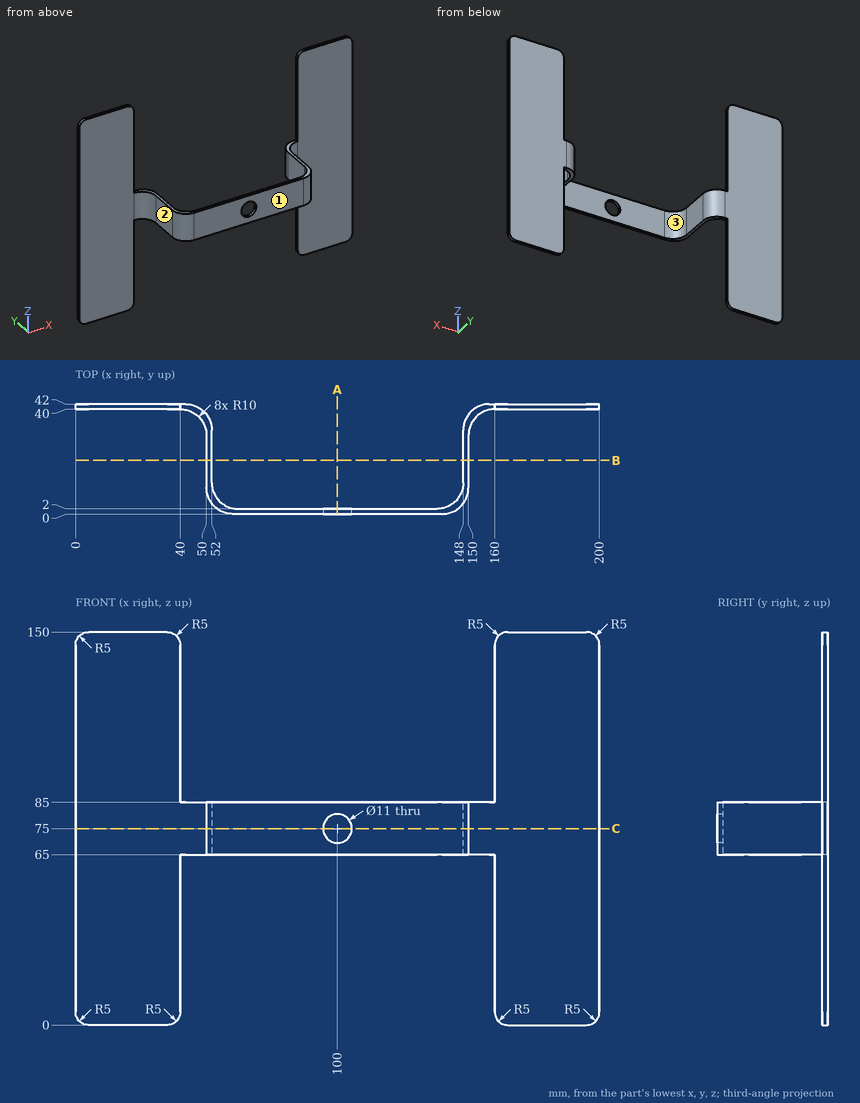
The figure shows three views and two pictorial views of one solid part (mm, origin at its lowest corner). Answer the questions. A direction names the side the tool comes from. Give positions to 0.01 mm unless a question says otherwise; leave off trailing zeros. Write each loop counter-clockwise with the first axis right and the second up, starting at its lowest first coordinate (ties: lowest second). Pieces come first, ordered by that corner, then holes. Notation, with made-up numbers: (87.5, 61) -> (128.5, 61) arc R19 cw to (128.5, 67) -> close; hole circle Ø7 at (51.5, 76.5). An arc over 180 degrees is marked (long way). Use one line per item in the form item = value.
1) Each of these flat-tipped pins is pushed along its axis until it touches: P1, Ø6, axis at x = 108, z = 71, coming from the +Y side; P2, Ø10, axis at x = 59, z = 94, coming from the +Y side; P3, Ø1.6, axis at y = 40.5, z = 102, coming from the -X side; P4, Ø6, axis at y = 19.5, z = 77, coming from the +X side. Where does it stop, or does it pass through?
Result:
P1 = 2
P2 = through
P3 = 0
P4 = 150
2) Section C-C on z = 75 is taken. Write down the section's boundary in (x, y), plus the area to 3 significant figures.
Result:
outline = (0, 40) -> (40, 40) arc R10 cw to (50, 30) -> (50, 10) arc R10 ccw to (60, 0) -> (94.5, 0) -> (94.5, 2) -> (62, 2) arc R10 cw to (52, 12) -> (52, 32) arc R10 ccw to (42, 42) -> (0, 42) -> close; (105.5, 0) -> (140, 0) arc R10 ccw to (150, 10) -> (150, 30) arc R10 cw to (160, 40) -> (200, 40) -> (200, 42) -> (158, 42) arc R10 ccw to (148, 32) -> (148, 12) arc R10 cw to (138, 2) -> (105.5, 2) -> close
area = 538 mm²
3) Straight lines are drawn through the part: probe 1 along Z at (x, y) = (100, 0.9); probe 2 along X at (y, z) = (36.5, 78.5); probe 3 along Y at (x, z) = (182.5, 134.5). For each, find the intervals that lie inside material, in ascending order.
Result:
probe_1 = 65 to 69.5, 80.5 to 85
probe_2 = 47.6 to 50.93, 149.07 to 152.4
probe_3 = 40 to 42
4) A tool of negligible diameter and unlimited length cuts with its end or side. For the marked faces 1, 2 and 3, from which of +Z, -Z, +X, -X, +Y, -Y can it reach the whole face along a straight path? Write none if from no direction.
Result:
face_1 = +Z, -Z, +X, -X, -Y
face_2 = +Z, -Z, -X, -Y
face_3 = +Z, -Z, +Y
5) Section B-B on y = 20.5 is taken. Write down the section's boundary in (x, z), plus the area to 3 significant figures.
Result:
outline = (50, 65) -> (52, 65) -> (52, 85) -> (50, 85) -> close; (148, 65) -> (150, 65) -> (150, 85) -> (148, 85) -> close
area = 80.0 mm²
6) Section A-A on x = 100 is taken. Write down the section's boundary in (y, z), plus the area to 3 significant figures.
Result:
outline = (0, 65) -> (2, 65) -> (2, 69.5) -> (0, 69.5) -> close; (0, 80.5) -> (2, 80.5) -> (2, 85) -> (0, 85) -> close
area = 18.0 mm²
